The model under review builds one solid part; all positions refer to its coordinate system, in mm. Face numbers are marked on the shaded views. Round coordinates to 2 decimals unless told otherwise and drop trailing zeros. Write each loop counter-clockwise with the first axis right and the second up, starting at its lowest first coordinate (ties: lowest second). Pieces come first, ordered by that corner, then holes. Notation, with made-up numbers: M -15,80.25 L -1,80.25 A20 cw -1,113.25 Z; hole C -25,-4 d3. An arc over 180 degrees is marked long. One line per item, written item: value. Start each with the question number.
1) Take a section at C-C, the plane z = -13.5. Write out the cut boundary in (x, y).
2) Take a section at B-B, the plane y = -15. State how many separate pieces and enclosed holes the cut face has, and give its area (3 significant figures).
3) Mouldability with a two-part tool opening along Y and no side actions: class the marked faces 1, 2 and 3 as +Y half, -Y half, draft (parallel to the pull), parting line (faces both ways), or undercut.
4) Take a section at A-A, the plane z = 56.5. Write out the cut boundary in (x, y), and give its area (3 significant figures).
5) Take a section at D-D, the plane z = 14.5. Write out the cut boundary in (x, y).
6) For P1, Ø6, axis at x = -40, z = 28, coming from the -Y side; P2, Ø1.5, axis at y = -12, z = 43, coming from the +X side; P3, Ø5, axis at x = -38.5, z = -23.5, coming from the -Y side, all flat-tipped, find the tip position at first contact; note any pin that passes through.
7) Wall thickness on probe 1 along X at (y, z) = (0, 36); probe 2 along Z at (x, y) = (-39, -14.5); probe 3 along Z at (x, y) = (-50.5, -8): over which ranges is each line inside the solid? List them lowest first.
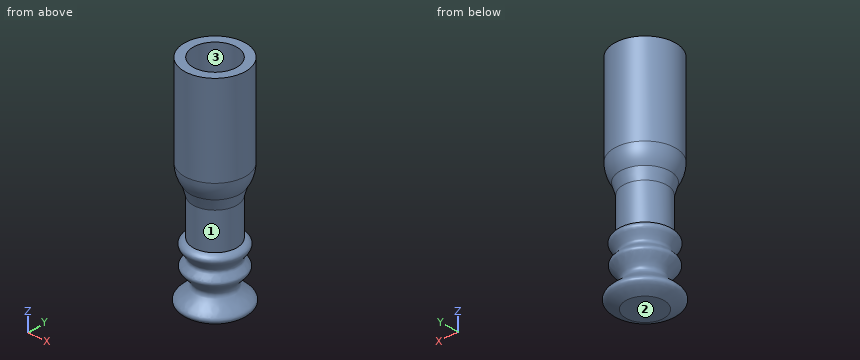
from build123d import *


with BuildPart() as f1:
    # F0 (on Front) → F1 (revolve)
    with BuildSketch(Plane.XZ):
        with BuildLine():
            Line((-26.0182898492, 5.7244500987), (-24.3058805849, 11.7220224141))
            ThreePointArc((-24.3058805849, 11.7220224141), (-21.979591378, 16.3704601156), (-21.1788231733, 21.506447345))
            Line((-21.1788231733, 21.506447345), (-21.1788231733, 71.7382878065))
            Line((-21.1788231733, 71.7382878065), (-26.0182898492, 71.7382878065))
            Line((-26.0182898492, 71.7382878065), (-26.0182898492, 21.506447345))
            Line((-26.0182898492, 21.506447345), (-38.0498692393, 21.506447345))
            Line((-38.0498692393, 21.506447345), (-38.0498692393, -48.8782897592))
            Line((-38.0498692393, -48.8782897592), (-27.5222361088, -48.8782897592))
            add(Edge.make_bspline(
                [(-26.0182898492, -14.5882898942), (-23.305044616, -15.5524146318), (-21.4055576786, -18.0960485839), (-28.7584352596, -23.8301011929), (-19.316895301, -28.1156810521), (-33.3537949524, -35.970450647), (-15.7526736038, -44.0802165493), (-23.6606204493, -47.2933194957), (-27.5222361088, -48.8782897592)],
                knots=[0, 0, 0, 0, 0.1337832997, 0.2873849573, 0.4311076344, 0.6155235378, 0.8189732636, 1, 1, 1, 1], degree=3))
            Line((-26.0182898492, -14.5882898942), (-26.0182898492, 5.7244500987))
        make_face()
    revolve(axis=Axis((-38.0498692393, 0, -13.6859212071), (0, 0, -1)))


solid = f1.part
Checked values:
1. outline: C -38.05,0 d24.06
2. separate pieces: 4
2. enclosed holes: 0
2. area: 957 mm2
3. face 1: parting line
3. face 2: draft
3. face 3: undercut
4. outline: C -38.05,0 d33.74; hole C -38.05,0 d24.06
4. area: 439 mm2
5. outline: C -38.05,0 d30.69
6. P1: stops at y = -16.87
6. P2: stops at x = -25.48
6. P3: stops at y = -13.82
7. probe 1: x = -54.92 to -50.08, -26.02 to -21.18
7. probe 2: z = -47.12 to -40.7, -29.39 to -26.79, -19.11 to -15.94, 12.93 to 71.74
7. probe 3: z = -46.99 to -40.91, -28.94 to -27.2, -18.68 to -16.24, 13.41 to 71.74
